Can you work these out from the model? Positions are in its coordinate system, mm. Give positions to 0.01 mm unless a question says otherwise; leave off trailing zeros. Loops run counter-clockwise (first coordinate to the right, second up) from the corner with the lowest first, then second, coordinate; pieces in that order, holes last. Notation, with made-up numbers: (-38.75, 49.5) - (-2.75, 49.5) arc R19 ccw to (-2.75, 82.5) - close; hole circle Ø11 at (70, 80.25). An arc over 180 degrees is marked (long way). Answer as a JSON object with one key per item and string values.
```python
from build123d import *

# Parameters (mm, degrees)
SKETCH1_W           = 250
SKETCH1_H           = 170
BOSS_EXTRUDE1_DEPTH = 2.5
SKETCH2_R           = 3.75
CUT_EXTRUDE1_DEPTH  = 3.5
FILLET1_R           = 8
SKETCH4_W           = 40
SKETCH4_H           = 50
BOSS_EXTRUDE2_DEPTH = 15


with BuildPart() as part:
    # Sketch1 → Boss-Extrude1 (new body)
    with BuildSketch(Plane(origin=(0, 0, 0), x_dir=(1, 0, 0), z_dir=(0, 1, 0))):
        Rectangle(SKETCH1_W, SKETCH1_H)
    extrude(amount=BOSS_EXTRUDE1_DEPTH)

    # Sketch2 → Cut-Extrude1 (cut, through all)
    with BuildSketch(Plane(origin=(0, 2.5, 0), x_dir=(1, 0, 0), z_dir=(0, 1, 0))):
        with Locations((-115, 36)):
            Circle(SKETCH2_R)
        with Locations((-115, -36)):
            Circle(SKETCH2_R)
        with Locations((115, -36)):
            Circle(SKETCH2_R)
        with Locations((115, 36)):
            Circle(SKETCH2_R)
    extrude(amount=-CUT_EXTRUDE1_DEPTH, mode=Mode.SUBTRACT)

    # Fillet1
    fillet1_edges = [part.edges().sort_by_distance(p)[0] for p in [
        (-125, 1.25, -85),
        (125, 1.25, -85),
        (125, 1.25, 85),
        (-125, 1.25, 85),
    ]]
    fillet(fillet1_edges, radius=FILLET1_R)

    # Sketch4 → Boss-Extrude2 (add)
    with BuildSketch(Plane.XZ):
        with Locations((0, 16)):
            Rectangle(SKETCH4_W, SKETCH4_H)
    extrude(amount=BOSS_EXTRUDE2_DEPTH)


solid = part.part
```
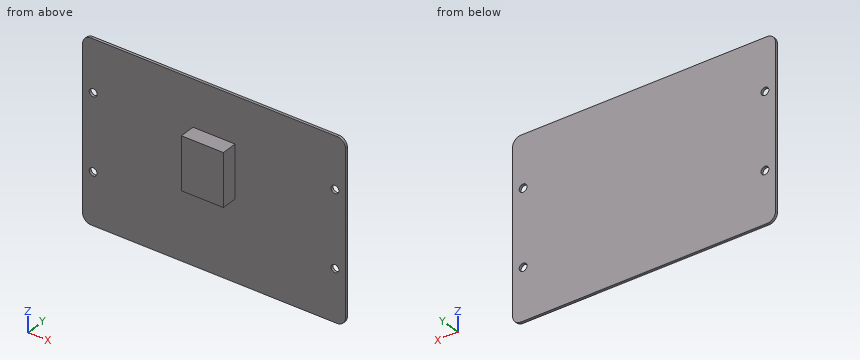
1) Imagine slicing it at D-D on z = -36. Write out the boundary of the cut face in (x, y).
Check sheet entries:
{"outline": "(-125, 0) - (-118.75, 0) - (-118.75, 2.5) - (-125, 2.5) - close; (-111.25, 0) - (111.25, 0) - (111.25, 2.5) - (-111.25, 2.5) - close; (118.75, 0) - (125, 0) - (125, 2.5) - (118.75, 2.5) - close"}
2) I need wall thicknesses on L1, parallel to Z at x = -115, y = 1.95; L2, parallel to X at y = 1.25, z = 36; L3, parallel to Y at x = -75, z = -57. Which ranges of each line are inside material? Lowest first, please.
Check sheet entries:
{"L1": "-85 to -39.75, -32.25 to 32.25, 39.75 to 85", "L2": "-125 to -118.75, -111.25 to 111.25, 118.75 to 125", "L3": "0 to 2.5"}
3) Imagine slicing it at C-C on z = 2.5. Write out the boundary of the cut face in (x, y), and give its area (4 significant figures).
Check sheet entries:
{"outline": "(-125, 0) - (-20, 0) - (-20, -15) - (20, -15) - (20, 0) - (125, 0) - (125, 2.5) - (-125, 2.5) - close", "area": "1,225 mm2"}
4) I'm going to push flat-ended pins straight in: P1, Ø10, axis at x = -62.5, y = -2.5, coming from the +Z side; P2, Ø7.5, axis at x = 3, y = -6.5, coming from the +Z side; P3, Ø6, axis at x = -115, z = -36, coming from the +Y side; P4, Ø7.5, axis at x = 4, y = -10.5, coming from the -Z side. Where does each tip first touch, or does it pass through?
Check sheet entries:
{"P1": "z = 85", "P2": "z = 41", "P3": "through", "P4": "z = -9"}
5) Imagine slicing it at A-A on z = 36. Write out the boundary of the cut face in (x, y), and give its area (3 significant figures).
Check sheet entries:
{"outline": "(-125, 0) - (-118.75, 0) - (-118.75, 2.5) - (-125, 2.5) - close; (-111.25, 0) - (-20, 0) - (-20, -15) - (20, -15) - (20, 0) - (111.25, 0) - (111.25, 2.5) - (-111.25, 2.5) - close; (118.75, 0) - (125, 0) - (125, 2.5) - (118.75, 2.5) - close", "area": "1,190 mm2"}
6) Imagine slicing it at B-B on x = 9. Write out the boundary of the cut face in (y, z).
Check sheet entries:
{"outline": "(-15, -9) - (0, -9) - (0, -85) - (2.5, -85) - (2.5, 85) - (0, 85) - (0, 41) - (-15, 41) - close"}
